Here's how the part is built. I have some questions about the finished solid (model axes, mm). A direction names the side the tool comes from. Give positions to 0.01 mm unless a question says otherwise; leave off trailing zeros. Loops run counter-clockwise (first coordinate to the right, second up) from the corner with the lowest first, then second, coordinate; pieces in that order, holes last. Notation, with made-up numbers: (71.25, 46.5) - (79.25, 46.5) arc R11 cw to (79.25, 65.5) - close; hole circle Ø1 at (-34, 15). An arc over 180 degrees is marked (long way). Return JSON: item names as keys, results as strings. Group by question number.
(1) If we mould it in two halves opening along Z, with no side actions, what happens to faces 1 (the cylindrical face through (-1.725, 2.348, 7.644)), 2 (the cylindrical face through (0.18, 6.12, 1.43)), 3 (the cylindrical face through (-1.725, 17.169, -2.348)), 4 (the cylindrical face through (-1.725, 2.348, 26.694))? For each: released by +Z, released by -Z, zero draft, split by the parting line, or undercut.
(2) For P1, Ø6, axis at x = 0, z = 28.575, coming from the +Y side; P2, Ø8, axis at x = 0, z = 47.625, coming from the -Y side; P3, Ø6.5, axis at x = 5.5, y = 21.5, coming from the +Z side; P4, Ø1, axis at x = 4, y = 7, coming from the +Z side, each with a flat end and sliding along its axis, tell me the tip position at first contact or that it passes through.
(3) If we section it at B-B (z = 48): Please give me the cut outline in (x, y) (1 decimal).
(4) If we section it at A-A (x = 0): State how many separate pieces and enclosed holes the cut face has, then the cut area to 3 significant figures.
(5) On a 3-axis mill with a long thin cutter (end or side, diameter ignored), from which of +Z, -Z, +X, -X, +Y, -Y can I reach the whole of each face in a straight line? I mean faces 5 (the flat face through (3, 4.762, 28)), 6 (the flat face through (3, 21, -4.762)). Say none if no direction works.
(6) I need wall thicknesses on probe 1 along Z at (x, y) = (0, 1.9); probe 2 along Z at (x, y) = (0.5, 4.5); probe 3 along Y at (x, z) = (-10, 36.5). Which ranges of each line are inside material? Lowest first, please. Write a range as [from, to].
(7) If we section it at C-C (z = 14): Please give me the cut outline in (x, y).
Autodesk Inventor part; units mm, degrees
ref_plane "YZ Plane" through (0, 0, 0) normal (1, 0, 0) x (0, 1, 0)
ref_plane "XZ Plane" through (0, 0, 0) normal (0, 1, 0) x (-1, 0, 0)
ref_plane "XY Plane" through (0, 0, 0) normal (0, 0, 1) x (1, 0, 0)
sketch "Sketch1" plane through (0, 0, 0) normal (0, 0, 1) x (1, 0, 0)
  line L0 (-17.78, 0) -> (17.78, 0) construction
  line L1 (-12.7, 0) -> (12.7, 0)
  line L2 (12.7, 0) -> (12.7, 19.05)
  arc A0 (12.7, 19.05) -> (-12.7, 19.05) centre (0, 19.05) ccw
  line L3 (-12.7, 19.05) -> (-12.7, 0)
  point P0 (0, 0)
  dimension "d0" = 25.4
  dimension "d1" = 19.05
extrude "Plate1" add sketch "Sketch1" against normal blind 4.7625
sketch "Sketch2" plane through (12.7, 4.7625, -4.7625) normal (0, -1, 0) x (1, 0, 0)
  line L0 (-25.4, 0) -> (0, 0)
  line L1 (0, 0) -> (0, 57.15)
  line L2 (0, 57.15) -> (-25.4, 57.15)
  line L3 (-25.4, 57.15) -> (-25.4, 0)
edge flange "Flange1" height 57.15 angle 90 thickness 4.7625 bend radius 4.7625 thickness toward (0, -1, 0) relief tear relief width 4.7625 relief depth 2.3813 edges at (0, 0, 0) wall of the first edge with corners at (-12.7, 4.7625, -4.7625) (12.7, 4.7625, -4.7625) (12.7, 4.7625, 52.3875) (-12.7, 4.7625, 52.3875)
bend "Bend1"
corner "Corner1"
sketch "Sketch3" plane through (0, 0, -4.7625) normal (0, 0, -1) x (-1, 0, 0)
  arc A0 (12.7, 19.05) -> (-12.7, 19.05) centre (0, 19.05) ccw construction
  point P0 (0, 0)
hole "Hole1" at (0, 19.05, -4.7625) direction (0, 0, 1) diameter 5.1054 end through all
sketch "Sketch4" plane through (-12.7, 4.7625, 52.3875) normal (0, 1, 0) x (1, 0, 0)
  line L0 (25.4, 47.625) -> (0, 47.625) construction
  line L1 (0, 47.625) -> (0, 0) construction
  line L2 (0, 0) -> (25.4, 0) construction
  line L3 (25.4, 47.625) -> (25.4, 0) construction
  line L4 (0, 0) -> (25.4, 47.625) construction
  line L5 (12.7, 4.7625) -> (12.7, 42.8625) construction
  point P0 (12.7, 52.3875)
  point P1 (12.7, 23.8125)
  dimension "d22" = 38.1
hole "Hole2" at (0, 4.7625, 47.625) at (0, 4.7625, 28.575) at (0, 4.7625, 9.525) direction (0, -1, 0) diameter 5.1054 end through all
fillet "Corner Round1" radius 6.35 2 edges at (-12.7, 2.3812, 52.3875) (12.7, 2.3812, 52.3875)
equation "\"d20\" = Thickness"
equation "\"d4\" = Thickness"
equation "\"d5\" = BendReliefWidth"
equation "\"d6\" = BendReliefDepth"
equation "\"d7\" = MinimumRemnant"
equation "\"d8\" = TransitionRadius"
equation "\"d11\" = BendRadius"
equation "\"d12\" = CornerReliefSize"
equation "\"d13\" = GapSize"
equation "\"d14\" = JacobiRadiusSize"
equation "\"BendRadius\" = Thickness"
equation "\"BendReliefWidth\" = Thickness"
equation "\"BendReliefDepth\" = 0.5 * Thickness"
equation "\"CornerReliefSize\" = 4 * Thickness"
equation "\"MinimumRemnant\" = 2 * Thickness"
equation "\"TransitionRadius\" = BendRadius"
equation "\"JacobiRadiusSize\" = BendRadius"
equation "\"GapSize\" = Thickness"
properties part number "MOUNT,KICKER"
Values:
{
 "1": {"face 1": "undercut", "face 2": "released by +Z", "face 3": "zero draft", "face 4": "undercut"},
 "2": {"P1": "y = 4.76", "P2": "y = 0", "P3": "z = 0", "P4": "z = 1.08"},
 "3": {"outline": "(-12.4, 0) - (-2.5, 0) - (-2.5, 4.8) - (-12.4, 4.8) - close; (2.5, 0) - (12.4, 0) - (12.4, 4.8) - (2.5, 4.8) - close"},
 "4": {"separate pieces": "5", "enclosed holes": "0", "area": "289 mm2"},
 "5": {"face 5": "+Z, +X, -X, +Y", "face 6": "-Z, +X, -X, +Y, -Y"},
 "6": {"probe 1": "[-0.95, 6.97], [12.08, 26.02], [31.13, 45.07], [50.18, 52.39]", "probe 2": "[-3.33, 7.02], [12.03, 26.07], [31.08, 45.12], [50.13, 52.39]", "probe 3": "[0, 4.76]"},
 "7": {"outline": "(-12.7, 0) - (12.7, 0) - (12.7, 4.76) - (-12.7, 4.76) - close"}
}
